```python
from build123d import *

# Parameters (mm, degrees)
BASE_FLANGE1_DEPTH = 654.05
SKETCH6_R          = 21.9075
CUT_EXTRUDE1_DEPTH = 3.175
SKETCH7_R          = 2.4257
CUT_EXTRUDE2_DEPTH = 683.89076222
SKETCH8_R          = 2.4257
CUT_EXTRUDE3_DEPTH = 683.89076222
SKETCH9_R          = 2.4257
CUT_EXTRUDE4_DEPTH = 683.89076222
FILLET1_R          = 3.175
SKETCH10_W         = 152.4
SKETCH10_H         = 61.9125
CUT_EXTRUDE6_DEPTH = 683.89076222
FILLET2_R          = 3.175


# Sheet-metal steps are written as plain solids
with BuildPart() as part:
    # Sketch1 → Base-Flange1 (new body)
    with BuildSketch(Plane(origin=(0, 0, 0), x_dir=(0, 0, -1), z_dir=(1, 0, 0))):
        with BuildLine():
            Line((0, 0), (146.05, 0))
            ThreePointArc((146.05, 0), (150.540128061, 1.859871939), (152.4, 6.35))
            Line((152.4, 6.35), (152.4, 117.475))
            ThreePointArc((152.4, 117.475), (150.540128061, 121.965128061), (146.05, 123.825))
            Line((146.05, 123.825), (0, 123.825))
            Line((0, 123.825), (0, 120.65))
            Line((0, 120.65), (146.05, 120.65))
            ThreePointArc((146.05, 120.65), (148.29506403, 119.72006403), (149.225, 117.475))
            Line((149.225, 117.475), (149.225, 6.35))
            ThreePointArc((149.225, 6.35), (148.29506403, 4.10493597), (146.05, 3.175))
            Line((146.05, 3.175), (0, 3.175))
            Line((0, 3.175), (0, 0))
        make_face()
    extrude(amount=BASE_FLANGE1_DEPTH)

    # Sketch6 → Cut-Extrude1 (cut)
    with BuildSketch(Plane(origin=(0, 123.825, 0), x_dir=(1, 0, 0), z_dir=(0, 1, 0))):
        with Locations(Location((234.95, 46.0375, 0), (0, 0, 270))):
            Circle(SKETCH6_R)
    extrude(amount=-CUT_EXTRUDE1_DEPTH, mode=Mode.SUBTRACT)

    # Sketch7 → Cut-Extrude2 (cut, through all)
    with BuildSketch(Plane(origin=(0, 123.825, 0), x_dir=(1, 0, 0), z_dir=(0, 1, 0))):
        with Locations(Location((234.95, 12.2555, 0), (0, 0, 270))):
            Circle(SKETCH7_R)
        with Locations(Location((234.95, 79.8195, 0), (0, 0, 270))):
            Circle(SKETCH7_R)
        with Locations(Location((209.55, 12.2555, 0), (0, 0, 270))):
            Circle(SKETCH7_R)
        with Locations(Location((260.35, 12.2555, 0), (0, 0, 270))):
            Circle(SKETCH7_R)
        with Locations(Location((260.35, 79.8195, 0), (0, 0, 270))):
            Circle(SKETCH7_R)
        with Locations(Location((209.55, 79.8195, 0), (0, 0, 270))):
            Circle(SKETCH7_R)
    cut_extrude2 = extrude(amount=-CUT_EXTRUDE2_DEPTH, mode=Mode.SUBTRACT)

    # Sketch8 → Cut-Extrude3 (cut, through all)
    with BuildSketch(Plane(origin=(0, 123.825, 0), x_dir=(1, 0, 0), z_dir=(0, 1, 0))):
        with Locations(Location((644.525, 12.7, 0), (0, 0, 270))):
            Circle(SKETCH8_R)
        with Locations(Location((644.525, 71.4375, 0), (0, 0, 270))):
            Circle(SKETCH8_R)
        with Locations(Location((644.525, 130.175, 0), (0, 0, 270))):
            Circle(SKETCH8_R)
        with Locations(Location((9.525, 130.175, 0), (0, 0, 270))):
            Circle(SKETCH8_R)
        with Locations(Location((9.525, 71.4375, 0), (0, 0, 270))):
            Circle(SKETCH8_R)
        with Locations(Location((9.525, 12.7, 0), (0, 0, 270))):
            Circle(SKETCH8_R)
    extrude(amount=-CUT_EXTRUDE3_DEPTH, mode=Mode.SUBTRACT)

    # Sketch9 → Cut-Extrude4 (cut, through all)
    with BuildSketch(Plane(origin=(0, 0, -152.4), x_dir=(-1, 0, 0), z_dir=(0, 0, -1))):
        with Locations((-644.525, 74.6125)):
            Circle(SKETCH9_R)
        with Locations((-644.525, 49.2125)):
            Circle(SKETCH9_R)
        with Locations((-9.525, 49.2125)):
            Circle(SKETCH9_R)
        with Locations((-9.525, 74.6125)):
            Circle(SKETCH9_R)
        with Locations((-644.525, 100.0125)):
            Circle(SKETCH9_R)
        with Locations((-644.525, 23.8125)):
            Circle(SKETCH9_R)
        with Locations((-9.525, 23.8125)):
            Circle(SKETCH9_R)
        with Locations((-9.525, 100.0125)):
            Circle(SKETCH9_R)
    extrude(amount=-CUT_EXTRUDE4_DEPTH, mode=Mode.SUBTRACT)

    # Fillet1
    fillet1_edges = [part.edges().sort_by_distance(p)[0] for p in [
        (0, 1.5875, 0),
        (0, 122.2375, 0),
        (654.05, 1.5875, 0),
        (654.05, 122.2375, 0),
    ]]
    fillet(fillet1_edges, radius=FILLET1_R)

    # Sketch10 → Cut-Extrude6 (cut, through all)
    with BuildSketch(Plane(origin=(654.05, 0, 0), x_dir=(0, 0, -1), z_dir=(1, 0, 0))):
        with Locations((76.2, 92.86875)):
            Rectangle(SKETCH10_W, SKETCH10_H)
    extrude(amount=-CUT_EXTRUDE6_DEPTH, mode=Mode.SUBTRACT)

    # Fillet2
    fillet2_edges = [part.edges().sort_by_distance(p)[0] for p in [
        (654.05, 61.9125, -150.8125),
        (0, 61.9125, -150.8125),
    ]]
    fillet(fillet2_edges, radius=FILLET2_R)

    # Mirror1: Cut-Extrude2 across plane
    add(cut_extrude2.mirror(Plane(origin=(327.025, 0, 0), x_dir=(0, 0, 1), z_dir=(1, 0, 0))), mode=Mode.SUBTRACT)


solid = part.part
```
Geometry check sheet. Reference: the model listing, model coordinates, mm. A direction names the side the tool comes from. Coordinates: 2 decimals unless noted, no trailing zeros. Order: outer loops, then holes, each group sorted by start corner. A loop starts at its lowest first (then second) coordinate and runs counter-clockwise, first axis right, second up.
Q1. Tool access check on faces 1 (the face through (322, 35, -149.225)), 2 (the face through (0, 1, -111)). Record the directions out of +Z, -Z, +X, -X, +Y, -Y that give a thin tool (end or side, any length) a straight path to the whole face; none if there is none.
Reply:
face 1: +Z, +X, -X, +Y
face 2: +Z, -Z, -X, +Y, -Y
Q2. Sectioned sample at B-B on z = -96. Record the cut outline in (x, y) (3 decimals), and give its area (3 significant figures).
Reply:
outline: (0, 0) - (654.05, 0) - (654.05, 3.175) - (0, 3.175) - close
area: 2,080 mm2
Q3. Thickness scan on probe 1 along Z at (x, y) = (419.1, 0.9); probe 2 along Y at (x, z) = (69.5, -104) (3 decimals); probe 3 along Z at (x, y) = (556, 30.5) (3 decimals). Record the ranges inside material, lowest first.
Reply:
probe 1: z = -149.31 to -82.25, -77.39 to -14.68, -9.83 to 0
probe 2: y = 0 to 3.175
probe 3: z = -152.4 to -149.225
Q4. Depth check by flat-ended pin: pin 1 Ø4 at (x, y) = (150.5, 42.5) entering from +Z (3 decimals); pin 2 Ø1 at (x, z) = (488, -94) entering from +Y (3 decimals). Enter the tip coordinate at first touch or a pass-through.
Reply:
pin 1: stops at z = -149.225
pin 2: stops at y = 3.175
Q5. Sectioned sample at C-C on y = 14. Record the cut outline in (x, z) (3 decimals), and give its area (3 significant figures).
Reply:
outline: (0, -152.4) - (654.05, -152.4) - (654.05, -149.225) - (0, -149.225) - close
area: 2,080 mm2
